from build123d import *

# Parameters (mm, degrees)
F0_R     = 3.302
F1_DEPTH = 3.175


with BuildPart() as f1:
    # F0 (on Top) → F1 (new body)
    with BuildSketch(Plane.XY):
        with BuildLine():
            Line((-5.260512, 63.5), (-47.080256, 21.680256))
            ThreePointArc((-47.080256, 21.680256), (-49.83327, 7.83992), (-38.1, 0))
            Line((-38.1, 0), (-12.7, 0))
            ThreePointArc((-12.7, 0), (-3.719744, 3.719744), (0, 12.7))
            Line((0, 12.7), (0, 63.5))
            Line((0, 63.5), (-5.260512, 63.5))
        make_face()
        with Locations((-38.1, 12.7)):
            Circle(F0_R, mode=Mode.SUBTRACT)
        with Locations((-12.7, 12.7)):
            Circle(F0_R, mode=Mode.SUBTRACT)
    extrude(amount=F1_DEPTH)


solid = f1.part
Input: part model. Units: mm. Frame: model coordinates. Give positions to 0.01 mm unless a question says otherwise; leave off trailing zeros. Order: outer loops, then holes, each group sorted by start corner. A loop starts at its lowest first (then second) coordinate and runs counter-clockwise, first axis right, second up. Notation, with made-up numbers: (-4, 69.5) - (4, 69.5) arc R32 ccw to (4, 104.5) - close; hole circle Ø3 at (37.5, 10.25). An arc over 180 degrees is marked (long way). Answer as a JSON object with one key per item and string values. Group by question number.
Q1. First-contact query: pin 1 Ø1.5 at (x, z) = (-17, 1.5) entering from +Y; pin 2 Ø8.5 at (x, y) = (-38.1, 12.7) entering from +Z (3 decimals). Flat tips, straight axial feed; report the tip coordinate or a pass-through.
Q2. Line query: probe 1 along Y at (x, z) = (-12.7, 1.75); probe 2 along Y at (x, z) = (-35.5, 1.5); probe 3 along X at (y, z) = (49.5, 3.05). Output: solid intervals per line, ascending.
Q3. Cut plane B-B, the plane y = 12. Output: boundary loops of the cut face in (x, z) (3 decimals), then the cut area to 3 significant figures.
Q4. Cut plane D-D, the plane y = 20.5. Output: boundary loops of the cut face in (x, z) (3 decimals), then the cut area to 3 significant figures.
Q5. Cut plane A-A, the plane z = 1.35. Output: boundary loops of the cut face in (x, y), then the cut area to 3 significant figures.
Q6. Cut plane C-C, the plane x = -14. Output: boundary loops of the cut face in (y, z) (3 decimals), then the cut area to 3 significant figures.
Q7. Mould query, pull axis X, two halves, no side actions, for faces 1 (the face through (-49.9, 8, 1.6)), 2 (the face through (-13.13, 15.974, 1.565)), 3 (the face through (-3, 63.5, 2)). Classes: pulls with the +X half, pulls with the -X half, needs draft (parallel to the pull), parting line crosses it, or undercut.
Results:
{
 "1": {"pin 1": "y = 52.51", "pin 2": "z = 3.175"},
 "2": {"probe 1": "0 to 9.4, 16 to 56.06", "probe 2": "0 to 10.66, 14.74 to 33.26", "probe 3": "-19.26 to 0"},
 "3": {"outline": "(-50.781, 0) - (-41.327, 0) - (-41.327, 3.175) - (-50.781, 3.175) - close; (-34.873, 0) - (-15.927, 0) - (-15.927, 3.175) - (-34.873, 3.175) - close; (-9.473, 0) - (-0.019, 0) - (-0.019, 3.175) - (-9.473, 3.175) - close", "area": "120 mm^2"},
 "4": {"outline": "(-48.122, 0) - (0, 0) - (0, 3.175) - (-48.122, 3.175) - close", "area": "153 mm^2"},
 "5": {"outline": "(-47.08, 21.68) arc R12.7 ccw to (-38.1, 0) - (-12.7, 0) arc R12.7 ccw to (0, 12.7) - (0, 63.5) - (-5.26, 63.5) - close; hole circle Ø6.6 at (-38.1, 12.7); hole circle Ø6.6 at (-12.7, 12.7)", "area": "2,050 mm^2"},
 "6": {"outline": "(0, 0) - (9.665, 0) - (9.665, 3.175) - (0, 3.175) - close; (15.735, 0) - (54.761, 0) - (54.761, 3.175) - (15.735, 3.175) - close", "area": "155 mm^2"},
 "7": {"face 1": "pulls with the -X half", "face 2": "undercut", "face 3": "needs draft"}
}
